Could you check a few things on this model? Use its own coordinates, in mm. Coordinates: 2 decimals unless noted, no trailing zeros. Write each loop counter-clockwise with the first axis right and the second up, starting at its lowest first coordinate (ties: lowest second). Pieces come first, ordered by that corner, then holes. Notation, with made-up numbers: M 73.5,-2.5 L 102.5,-2.5 A13 ccw 102.5,18.5 Z; hole C 32,30 d1. An arc over 180 degrees is marked long. Answer as CSV lines item,"result". Start each with the question number.
Item 1: If I drill on line 1 along Z through (x, y) = (-118, 15.25); line 2 along X through (y, z) = (9.5, 166.5); line 3 along Z through (x, y) = (62, 25.5), over which ranges is the centre line in solid material (lowest first)? Write a range as [from, to].
Item 2: I'm going to push flat-ended pins straight in: P1, Ø11, axis at x = -118, z = 119, coming from the -Y side; P2, Ø24, axis at x = -127, z = 166.5, coming from the -Y side. Where does each tip first touch, or does it pass through?
Item 3: Suppose I cut it at A-A, the plane z = -168. Write out the boundary of the cut face in (x, y).
Item 4: Suppose I cut it at C-C, the plane x = -62. Write out the boundary of the cut face in (y, z), and give its area (3 significant figures).
Item 5: Suppose I cut it at B-B, the plane y = 22. State how many separate pieces and enclosed holes the cut face has, and give its area (3 significant figures).
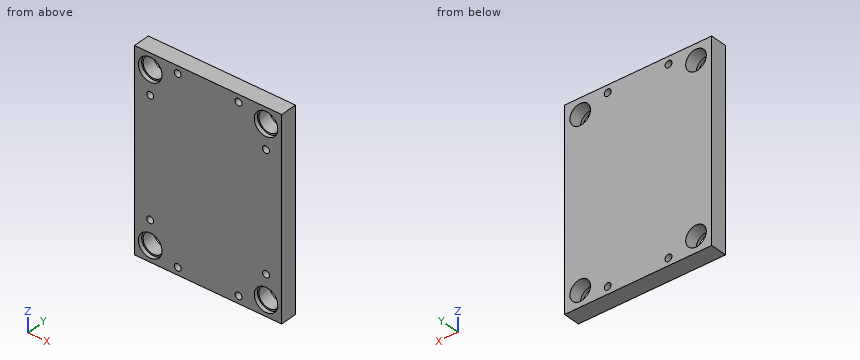
```python
from build123d import *

# Parameters (mm, degrees)
ESBO_O1_W                  = 300
ESBO_O1_H                  = 400
EXTRUS_O1_DEPTH            = 34
FURO_ROSCADO_DE_M161_D     = 14
FURO_ROSCADO_DE_M161_DEPTH = 28
FURO_ROSCADO_DE_M161_TIP   = 4.206024333
FURO1_D                    = 42
FURO1_CBORE_D              = 48
FURO1_CBORE_DEPTH          = 8
FURO2_D                    = 14
FURO2_DEPTH                = 100


with BuildPart() as part:
    # Esboço1 → Extrusão1 (new body)
    with BuildSketch(Plane(origin=(0, 0, 0), x_dir=(1, 0, 0), z_dir=(0, 1, 0))):
        Rectangle(ESBO_O1_W, ESBO_O1_H)
    extrude(amount=EXTRUS_O1_DEPTH)

    # Furo roscado de M161
    with Locations(Plane.XZ):
        with Locations((-118, 119), (118, 119), (-118, -119), (118, -119)):
            Hole(FURO_ROSCADO_DE_M161_D / 2, depth=FURO_ROSCADO_DE_M161_DEPTH)
            with Locations((0, 0, -(FURO_ROSCADO_DE_M161_DEPTH + FURO_ROSCADO_DE_M161_TIP / 2))):  # 118° drill point
                Cone(0, FURO_ROSCADO_DE_M161_D / 2, FURO_ROSCADO_DE_M161_TIP, mode=Mode.SUBTRACT)

    # Furo1 (through all)
    with Locations(Plane.XZ):
        with Locations((118, 168), (118, -168), (-118, -168), (-118, 168)):
            CounterBoreHole(FURO1_D / 2, FURO1_CBORE_D / 2, FURO1_CBORE_DEPTH)

    # Furo2
    with Locations(Plane.XZ):
        with Locations((-62, 185), (-62, -185), (62, 185), (62, -185)):
            Hole(FURO2_D / 2, depth=FURO2_DEPTH)


solid = part.part
```
Ans:
1,line 1,"z = [-200, -189], [-147, -126], [-112, 112], [126, 147], [189, 200]"
1,line 2,"x = [-150, -138.95], [-97.05, 97.05], [138.95, 150]"
1,line 3,"z = [-200, -192], [-178, 178], [192, 200]"
2,P1,"stops at y = 28.9"
2,P2,"stops at y = 8"
3,outline,"M -150,0 L -142,0 L -142,8 L -139,8 L -139,34 L -150,34 Z; M -97,8 L -94,8 L -94,0 L 94,0 L 94,8 L 97,8 L 97,34 L -97,34 Z; M 139,8 L 142,8 L 142,0 L 150,0 L 150,34 L 139,34 Z"
4,outline,"M 0,-200 L 34,-200 L 34,-192 L 0,-192 Z; M 0,-178 L 34,-178 L 34,178 L 0,178 Z; M 0,192 L 34,192 L 34,200 L 0,200 Z"
4,area,"12,600 mm^2"
5,separate pieces,"1"
5,enclosed holes,"12"
5,area,"113,000 mm^2"
